Geometry: final body of the model. Coordinates: model frame, mm. Face numbers are marked on the shaded views. A direction names the side the tool comes from. Give positions to 0.01 mm unless a question says otherwise; leave off trailing zeros. Write each loop counter-clockwise with the first axis right and the second up, starting at its lowest first coordinate (ties: lowest second). Pieces come first, ordered by that corner, then holes. Notation, with made-up numbers: (77.25, -32.75) - (110.25, -32.75) arc R12 ccw to (110.25, -9.75) - close; hole circle Ø4 at (45, -11). An arc over 180 degrees is marked (long way). Return JSON: item names as keys, results as strings.
from build123d import *

# Parameters (mm, degrees)
BOSS_EXTRUDE1_DEPTH = 38.1
FILLET1_R           = 2.54
FILLET2_R           = 10.16
CUT_EXTRUDE2_DEPTH  = 91.653895256
SKETCH3_R           = 1.5875
CUT_EXTRUDE3_DEPTH  = 91.653895256
SKETCH4_R           = 1.5875
CUT_EXTRUDE4_DEPTH  = 145.905274839


with BuildPart() as part:
    # Sketch1 → Boss-Extrude1 (new body)
    with BuildSketch(Plane.XY):
        with BuildLine():
            Line((-35.8775, -27.305), (38.4175, -27.305))
            ThreePointArc((38.4175, -27.305), (48.520288136, -23.120288136), (52.705, -13.0175))
            Line((52.705, -13.0175), (52.705, -1.5875))
            ThreePointArc((52.705, -1.5875), (54.099903955, 1.780096045), (57.4675, 3.175))
            Line((57.4675, 3.175), (62.23, 3.175))
            Line((62.23, 3.175), (62.23, 47.625))
            Line((62.23, 47.625), (52.705, 47.625))
            Line((52.705, 47.625), (52.705, 12.7))
            Line((52.705, 12.7), (43.18, 12.7))
            Line((43.18, 12.7), (43.18, -13.0175))
            ThreePointArc((43.18, -13.0175), (41.785096045, -16.385096045), (38.4175, -17.78))
            Line((38.4175, -17.78), (-35.8775, -17.78))
            ThreePointArc((-35.8775, -17.78), (-39.245096045, -16.385096045), (-40.64, -13.0175))
            Line((-40.64, -13.0175), (-40.64, 12.7))
            Line((-40.64, 12.7), (-50.165, 12.7))
            Line((-50.165, 12.7), (-59.69, 12.7))
            Line((-59.69, 12.7), (-69.215, 12.7))
            Line((-69.215, 12.7), (-69.215, 3.175))
            Line((-69.215, 3.175), (-50.165, 3.175))
            Line((-50.165, 3.175), (-50.165, -13.0175))
            ThreePointArc((-50.165, -13.0175), (-45.980288136, -23.120288136), (-35.8775, -27.305))
        make_face()
    extrude(amount=BOSS_EXTRUDE1_DEPTH)

    # Fillet1
    fillet1_edges = [part.edges().sort_by_distance(p)[0] for p in [
        (62.23, 3.175, 19.05),
    ]]
    fillet(fillet1_edges, radius=FILLET1_R)

    # Fillet2
    # the kernel refuses this fillet: 10.16 mm, written as the material it takes off along each edge
    with BuildSketch(Plane(origin=(-69.215, 3.175, -25.350342083), x_dir=(1, 0, 0), z_dir=(0, 0, 1))) as fillet2_piece_1:
        with BuildLine():
            CenterArc((10.140136833, 10.16), FILLET2_R, 183.583321698, 86.416678302)
            Line((0, 9.525), (-0.202802737, 9.5123))
            ThreePointArc((-0.202802737, 9.5123), (-0.2032, 4.7625), (-0.2032, 0))
            Line((-0.2032, 0), (0, -0.2032))
            Line((0, -0.2032), (10.140136833, -0.2032))
            Line((10.140136833, -0.2032), (10.140136833, 0))
        make_face()
    extrude(amount=88.800684167, mode=Mode.SUBTRACT)
    with BuildSketch(Plane(origin=(62.23, 47.625, -25.350342083), x_dir=(0, -1, 0), z_dir=(0, 0, 1))) as fillet2_piece_2:
        with BuildLine():
            CenterArc((10.140136833, -10.16), FILLET2_R, 90, 86.416678302)
            Line((0, -9.525), (-0.202802737, -9.5123))
            ThreePointArc((-0.202802737, -9.5123), (-0.2032, -4.7625), (-0.2032, 0))
            Line((-0.2032, 0), (0, 0.2032))
            Line((0, 0.2032), (10.140136833, 0.2032))
            Line((10.140136833, 0.2032), (10.140136833, 0))
        make_face()
    extrude(amount=88.800684167, mode=Mode.SUBTRACT)

    # Sketch2 → Cut-Extrude2 (cut, through all)
    with BuildSketch(Plane.XZ.offset(-3.175)):
        Polygon((-69.215, 19.05), (-69.215, 44.45), (-50.165, 44.45), align=None)
    extrude(amount=-CUT_EXTRUDE2_DEPTH, mode=Mode.SUBTRACT)

    # Sketch3 → Cut-Extrude3 (cut, through all)
    with BuildSketch(Plane.XZ.offset(-3.175)):
        with Locations((-64.144931583, 3.175)):
            Circle(SKETCH3_R)
        with Locations((-64.144931583, 11.317545611)):
            Circle(SKETCH3_R)
        with Locations((-64.144931583, 19.460091222)):
            Circle(SKETCH3_R)
    extrude(amount=-CUT_EXTRUDE3_DEPTH, mode=Mode.SUBTRACT)

    # Sketch4 → Cut-Extrude4 (cut, through all)
    with BuildSketch(Plane(origin=(62.23, 0, 0), x_dir=(0, 0, -1), z_dir=(1, 0, 0))):
        with Locations((-6.35, 42.554931583)):
            Circle(SKETCH4_R)
        with Locations((-19.05, 42.554931583)):
            Circle(SKETCH4_R)
        with Locations((-31.75, 42.554931583)):
            Circle(SKETCH4_R)
    extrude(amount=-CUT_EXTRUDE4_DEPTH, mode=Mode.SUBTRACT)


solid = part.part
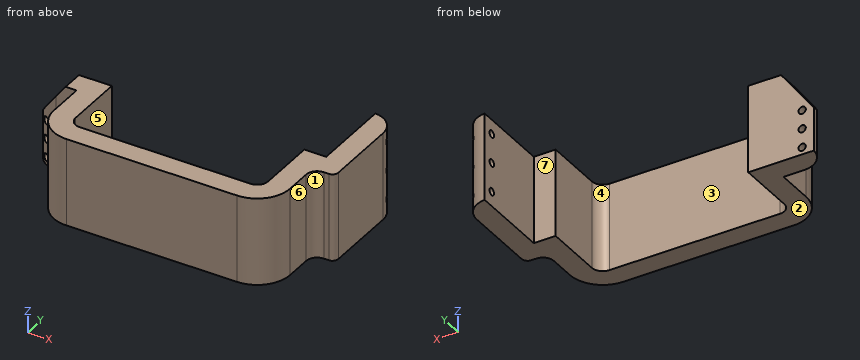
Q1. Section query B-B, the plane z = 6.35. Return the cut outline in (x, y) (1 decimal), plus the area to 3 significant figures.
Answer key:
{"outline": "(-69.2, 12.7) arc R10.2 ccw to (-59.1, 3.2) - (-50.2, 3.2) - (-50.2, -13) arc R14.3 ccw to (-35.9, -27.3) - (38.4, -27.3) arc R14.3 ccw to (52.7, -13) - (52.7, -1.6) arc R4.8 cw to (57.5, 3.2) - (59.7, 3.2) arc R2.5 ccw to (62.2, 5.7) - (62.2, 37.5) arc R10.2 ccw to (61.6, 41) - (52.7, 41) - (52.7, 12.7) - (43.2, 12.7) - (43.2, -13) arc R4.8 cw to (38.4, -17.8) - (-35.9, -17.8) arc R4.8 cw to (-40.6, -13) - (-40.6, 12.7) - close; (52.7, 44.1) - (59.7, 44.1) arc R10.2 ccw to (52.7, 47.6) - close", "area": "2,020 mm^2"}
Q2. Section query D-D, the plane z = 26.5. Return the cut outline in (x, y) (1 decimal).
Answer key:
{"outline": "(-63.6, 4.3) arc R10.2 ccw to (-59.1, 3.2) - (-50.2, 3.2) - (-50.2, -13) arc R14.3 ccw to (-35.9, -27.3) - (38.4, -27.3) arc R14.3 ccw to (52.7, -13) - (52.7, -1.6) arc R4.8 cw to (57.5, 3.2) - (59.7, 3.2) arc R2.5 ccw to (62.2, 5.7) - (62.2, 37.5) arc R10.2 ccw to (52.7, 47.6) - (52.7, 12.7) - (43.2, 12.7) - (43.2, -13) arc R4.8 cw to (38.4, -17.8) - (-35.9, -17.8) arc R4.8 cw to (-40.6, -13) - (-40.6, 12.7) - (-63.6, 12.7) - close"}
Q3. Section query C-C, the plane y = 20.5. Return the cut outline in (x, z) (3 decimals).
Answer key:
{"outline": "(52.705, 0) - (62.23, 0) - (62.23, 38.1) - (52.705, 38.1) - close"}
Q4. Section query A-A, the plane y = -10.5. Return the cut outline in (x, z) (3 decimals).
Answer key:
{"outline": "(-50.165, 0) - (-40.64, 0) - (-40.64, 38.1) - (-50.165, 38.1) - close; (43.18, 0) - (52.705, 0) - (52.705, 38.1) - (43.18, 38.1) - close"}
Q5. Mould query, pull axis X, two halves, no side actions, for the marked faces 1, 2, 3 and 4. Classes: pulls with the +X half, pulls with the -X half, needs draft (parallel to the pull), parting line crosses it, or undercut.
Answer key:
{"face 1": "pulls with the +X half", "face 2": "needs draft", "face 3": "undercut", "face 4": "undercut"}
Q6. Material intervals for probe 1 along X at (y, z) = (-5.5, 16.5) (3 decimals); probe 2 along X at (y, z) = (16, 16) (3 decimals); probe 3 along Y at (x, z) = (54.75, 31.75), sorted ascending. Write a range as [from, to].
Answer key:
{"probe 1": "x = [-50.165, -40.64], [43.18, 52.705]", "probe 2": "x = [52.705, 62.23]", "probe 3": "y = [2.32, 40.97], [44.14, 47.29]"}
Q7. Set-up query: the marked faces 5, 6 and 7. Return all of +Z, -Z, +X, -X, +Y, -Y with unobstructed straight access to the full face (end or side cutting, diameter ignored); none if empty.
Answer key:
{"face 5": "+Z, -Z, +Y", "face 6": "+Z, -Z, +X, -Y", "face 7": "+Z, -Z, -X, +Y"}
Q8. Pin query (flat end, axial travel): P1, Ø10.5, axis at y = 26.5, z = 27.5, coming from the -X side (3 decimals); P2, Ø2, axis at y = -11.5, z = 7.5, coming from the +X side (3 decimals); P3, Ø5, axis at y = -4.5, z = 11, coming from the -X side (3 decimals). Return the tip coordinate at first contact, or that it passes through.
Answer key:
{"P1": "stops at x = 52.705", "P2": "stops at x = 52.705", "P3": "stops at x = -50.165"}
